from build123d import *

# Parameters (mm, degrees)
BOSS_EXTRUDE1_DEPTH                             = 15
SKETCH2_W                                       = 60
SKETCH2_H                                       = 110
BOSS_EXTRUDE2_DEPTH                             = 5
SKETCH3_R                                       = 1.25
BOSS_EXTRUDE3_DEPTH                             = 4
SKETCH4_R                                       = 1.405
BOSS_EXTRUDE4_DEPTH                             = 1
CHAMFER1_SIZE                                   = 0.5
SKETCH5_W                                       = 1
SKETCH5_H                                       = 3.260897444
CUT_EXTRUDE1_DEPTH                              = 4
SKETCH7_R                                       = 1.25
BOSS_EXTRUDE5_DEPTH                             = 4
SKETCH8_R                                       = 1.405
BOSS_EXTRUDE6_DEPTH                             = 1
CHAMFER2_SIZE                                   = 0.5
SKETCH9_W                                       = 1
SKETCH9_H                                       = 4.099421272
SKETCH9_H_2                                     = 4.814063164
CUT_EXTRUDE2_DEPTH                              = 4
SKETCH10_R                                      = 1.25
BOSS_EXTRUDE7_DEPTH                             = 4
SKETCH11_R                                      = 1.405
BOSS_EXTRUDE8_DEPTH                             = 1
CHAMFER3_SIZE                                   = 0.5
SKETCH12_W                                      = 1
SKETCH12_H                                      = 3.78691003
CUT_EXTRUDE3_DEPTH                              = 4
SKETCH14_W                                      = 27
SKETCH14_H                                      = 64
BOSS_EXTRUDE9_DEPTH                             = 5
CUT_EXTRUDE6_DEPTH                              = 85.858706094
SKETCH15_R                                      = 1
BOSS_EXTRUDE10_DEPTH                            = 4
SKETCH16_R                                      = 1.175
BOSS_EXTRUDE11_DEPTH                            = 1
CHAMFER4_SIZE                                   = 0.5
SKETCH17_W                                      = 1
SKETCH17_H                                      = 3.189279986
CUT_EXTRUDE7_DEPTH                              = 4
SKETCH20_R                                      = 1
BOSS_EXTRUDE12_DEPTH                            = 4
SKETCH21_R                                      = 1.405
BOSS_EXTRUDE13_DEPTH                            = 1
CHAMFER5_SIZE                                   = 0.5
SKETCH23_W                                      = 1
SKETCH23_H                                      = 4.222684002
CUT_EXTRUDE8_DEPTH                              = 4
CUT_EXTRUDE9_DEPTH                              = 82.547532152
SKETCH26_W                                      = 5
SKETCH26_H                                      = 5
BOSS_EXTRUDE15_DEPTH                            = 30
BOSS_EXTRUDE16_DEPTH                            = 5
CSK_FOR_M4_FLAT_HEAD_MACHINE_SCREW2_D           = 4.5
CSK_FOR_M4_FLAT_HEAD_MACHINE_SCREW2_DEPTH       = 5
CSK_FOR_M4_FLAT_HEAD_MACHINE_SCREW2_CSINK_D     = 9.4
CSK_FOR_M4_FLAT_HEAD_MACHINE_SCREW2_CSINK_ANGLE = 90
CSK_FOR_M4_FLAT_HEAD_MACHINE_SCREW2_TIP         = 1.351936393


with BuildPart() as part:
    # Sketch1 → Boss-Extrude1 (new, symmetric)
    with BuildSketch(Plane.XY):
        Polygon((0, 0), (10, 0), (55, 2.358350068), (54.738678842, 7.344654806), (10, 5), (5, 5), (5, 24), (60, 24), (60, 29), (0, 29), align=None)
    extrude(amount=BOSS_EXTRUDE1_DEPTH, both=True)

    # Sketch2 → Boss-Extrude2 (add)
    with BuildSketch(Plane(origin=(0, 29, 0), x_dir=(1, 0, 0), z_dir=(0, 1, 0))):
        with Locations((30, 0)):
            Rectangle(SKETCH2_W, SKETCH2_H)
    extrude(amount=-BOSS_EXTRUDE2_DEPTH)

    # Sketch3 → Boss-Extrude3 (add)
    with BuildSketch(Plane(origin=(0, 29, 0), x_dir=(1, 0, 0), z_dir=(0, 1, 0))):
        with Locations(Location((54, -37, 0), (0, 0, 90))):
            Circle(SKETCH3_R)
    extrude(amount=BOSS_EXTRUDE3_DEPTH)

    # Sketch4 → Boss-Extrude4 (add)
    with BuildSketch(Plane(origin=(0, 33, 0), x_dir=(1, 0, 0), z_dir=(0, 1, 0))):
        with Locations(Location((54, -37, 0), (0, 0, 270))):
            Circle(SKETCH4_R)
    extrude(amount=BOSS_EXTRUDE4_DEPTH)

    # Chamfer1
    chamfer1_edges = [part.edges().sort_by_distance(p)[0] for p in [
        (54, 34, 35.595),
    ]]
    chamfer(chamfer1_edges, length=CHAMFER1_SIZE)

    # Sketch5 → Cut-Extrude1 (cut)
    with BuildSketch(Plane(origin=(0, 34, 0), x_dir=(1, 0, 0), z_dir=(0, 1, 0))):
        with Locations((54, -37)):
            Rectangle(SKETCH5_W, SKETCH5_H)
    extrude(amount=-CUT_EXTRUDE1_DEPTH, mode=Mode.SUBTRACT)

    # Sketch7 → Boss-Extrude5 (add)
    with BuildSketch(Plane(origin=(0, 29, 0), x_dir=(1, 0, 0), z_dir=(0, 1, 0))):
        with Locations(Location((54.3, 46, 0), (0, 0, 90))):
            Circle(SKETCH7_R)
        with Locations(Location((5.7, 40, 0), (0, 0, 90))):
            Circle(SKETCH7_R)
    extrude(amount=BOSS_EXTRUDE5_DEPTH)

    # Sketch8 → Boss-Extrude6 (add)
    with BuildSketch(Plane(origin=(0, 33, 0), x_dir=(1, 0, 0), z_dir=(0, 1, 0))):
        with Locations(Location((5.7, 40, 0), (0, 0, 270))):
            Circle(SKETCH8_R)
        with Locations(Location((54.3, 46, 0), (0, 0, 270))):
            Circle(SKETCH8_R)
    extrude(amount=BOSS_EXTRUDE6_DEPTH)

    # Chamfer2
    chamfer2_edges = [part.edges().sort_by_distance(p)[0] for p in [
        (5.7, 34, -41.405),
        (54.3, 34, -47.405),
    ]]
    chamfer(chamfer2_edges, length=CHAMFER2_SIZE)

    # Sketch9 → Cut-Extrude2 (cut)
    with BuildSketch(Plane(origin=(0, 34, 0), x_dir=(1, 0, 0), z_dir=(0, 1, 0))):
        with Locations((5.7, 40)):
            Rectangle(SKETCH9_W, SKETCH9_H)
        with Locations((54.3, 46)):
            Rectangle(SKETCH9_W, SKETCH9_H_2)
    extrude(amount=-CUT_EXTRUDE2_DEPTH, mode=Mode.SUBTRACT)

    # Sketch10 → Boss-Extrude7 (add)
    with BuildSketch(Plane(origin=(0, 29, 0), x_dir=(1, 0, 0), z_dir=(0, 1, 0))):
        with Locations(Location((6, -35, 0), (0, 0, 90))):
            Circle(SKETCH10_R)
    extrude(amount=BOSS_EXTRUDE7_DEPTH)

    # Sketch11 → Boss-Extrude8 (add)
    with BuildSketch(Plane(origin=(0, 33, 0), x_dir=(1, 0, 0), z_dir=(0, 1, 0))):
        with Locations(Location((6, -35, 0), (0, 0, 270))):
            Circle(SKETCH11_R)
    extrude(amount=BOSS_EXTRUDE8_DEPTH)

    # Chamfer3
    chamfer3_edges = [part.edges().sort_by_distance(p)[0] for p in [
        (6, 34, 33.595),
    ]]
    chamfer(chamfer3_edges, length=CHAMFER3_SIZE)

    # Sketch12 → Cut-Extrude3 (cut)
    with BuildSketch(Plane(origin=(0, 34, 0), x_dir=(1, 0, 0), z_dir=(0, 1, 0))):
        with Locations((6, -35)):
            Rectangle(SKETCH12_W, SKETCH12_H)
    extrude(amount=-CUT_EXTRUDE3_DEPTH, mode=Mode.SUBTRACT)

    # Sketch14 → Boss-Extrude9 (add)
    with BuildSketch(Plane(origin=(0, 29, 0), x_dir=(1, 0, 0), z_dir=(0, 1, 0))):
        with Locations((-13.5, 23)):
            Rectangle(SKETCH14_W, SKETCH14_H)
    extrude(amount=-BOSS_EXTRUDE9_DEPTH)

    # Sketch13 → Cut-Extrude6 (cut, through all)
    with BuildSketch(Plane.XZ.offset(-24)):
        Polygon((0, 15), (0, -15), (0, -55), (60, -55), (60, 55), (0, 55), align=None)
    extrude(amount=CUT_EXTRUDE6_DEPTH, mode=Mode.SUBTRACT)

    # Sketch15 → Boss-Extrude10 (add)
    with BuildSketch(Plane(origin=(0, 29, 0), x_dir=(1, 0, 0), z_dir=(0, 1, 0))):
        with Locations(Location((-23, -6.2, 0), (0, 0, 90))):
            Circle(SKETCH15_R)
        with Locations(Location((-4, -6.2, 0), (0, 0, 90))):
            Circle(SKETCH15_R)
    extrude(amount=BOSS_EXTRUDE10_DEPTH)

    # Sketch16 → Boss-Extrude11 (add)
    with BuildSketch(Plane(origin=(0, 33, 0), x_dir=(1, 0, 0), z_dir=(0, 1, 0))):
        with Locations(Location((-23, -6.2, 0), (0, 0, 270))):
            Circle(SKETCH16_R)
        with Locations(Location((-4, -6.2, 0), (0, 0, 270))):
            Circle(SKETCH16_R)
    extrude(amount=BOSS_EXTRUDE11_DEPTH)

    # Chamfer4
    chamfer4_edges = [part.edges().sort_by_distance(p)[0] for p in [
        (-23, 34, 5.025),
        (-4, 34, 5.025),
    ]]
    chamfer(chamfer4_edges, length=CHAMFER4_SIZE)

    # Sketch17 → Cut-Extrude7 (cut)
    with BuildSketch(Plane(origin=(0, 34, 0), x_dir=(1, 0, 0), z_dir=(0, 1, 0))):
        with Locations((-23, -6.2)):
            Rectangle(SKETCH17_W, SKETCH17_H)
        with Locations((-4, -6.2)):
            Rectangle(SKETCH17_W, SKETCH17_H)
    extrude(amount=-CUT_EXTRUDE7_DEPTH, mode=Mode.SUBTRACT)

    # Sketch20 → Boss-Extrude12 (add)
    with BuildSketch(Plane(origin=(0, 29, 0), x_dir=(1, 0, 0), z_dir=(0, 1, 0))):
        with Locations(Location((-23, 50.3, 0), (0, 0, 90))):
            Circle(SKETCH20_R)
        with Locations(Location((-4, 50.3, 0), (0, 0, 90))):
            Circle(SKETCH20_R)
    extrude(amount=BOSS_EXTRUDE12_DEPTH)

    # Sketch21 → Boss-Extrude13 (add)
    with BuildSketch(Plane(origin=(0, 33, 0), x_dir=(1, 0, 0), z_dir=(0, 1, 0))):
        with Locations(Location((-23, 50.3, 0), (0, 0, 270))):
            Circle(SKETCH21_R)
        with Locations(Location((-4, 50.3, 0), (0, 0, 270))):
            Circle(SKETCH21_R)
    extrude(amount=BOSS_EXTRUDE13_DEPTH)

    # Chamfer5
    chamfer5_edges = [part.edges().sort_by_distance(p)[0] for p in [
        (-23, 34, -51.705),
        (-4, 34, -51.705),
    ]]
    chamfer(chamfer5_edges, length=CHAMFER5_SIZE)

    # Sketch23 → Cut-Extrude8 (cut)
    with BuildSketch(Plane(origin=(0, 34, 0), x_dir=(1, 0, 0), z_dir=(0, 1, 0))):
        with Locations((-23, 50.3)):
            Rectangle(SKETCH23_W, SKETCH23_H)
        with Locations((-4, 50.3)):
            Rectangle(SKETCH23_W, SKETCH23_H)
    extrude(amount=-CUT_EXTRUDE8_DEPTH, mode=Mode.SUBTRACT)

    # Sketch18 → Cut-Extrude9 (cut, through all)
    with BuildSketch(Plane(origin=(0, 29, 0), x_dir=(1, 0, 0), z_dir=(0, 1, 0))):
        Polygon((-22, 45.3), (0.7, 45.3), (0.7, 35), (10.7, 35), (10.7, 50), (49.3, 50), (49.3, 41), (55, 41), (55, -32), (49, -32), (49, -42), (55, -42), (55, -50), (6, -50), (6, -40), (11, -40), (11, -30), (5, -30), (5, -1.2), (-22, -1.2), align=None)
    extrude(amount=-CUT_EXTRUDE9_DEPTH, mode=Mode.SUBTRACT)

    # Sketch26 → Boss-Extrude15 (add)
    with BuildSketch(Plane.XZ.offset(-24)):
        with Locations((2.5, 52.5)):
            Rectangle(SKETCH26_W, SKETCH26_H)
        with Locations((57.5, 52.5)):
            Rectangle(SKETCH26_W, SKETCH26_H)
        with Locations((57.5, -52.5)):
            Rectangle(SKETCH26_W, SKETCH26_H)
        with Locations((-24.5, -52.5)):
            Rectangle(SKETCH26_W, SKETCH26_H)
        with Locations((-24.5, 6.5)):
            Rectangle(SKETCH26_W, SKETCH26_H)
    extrude(amount=BOSS_EXTRUDE15_DEPTH)

    # Sketch27 → Boss-Extrude16 (add)
    with BuildSketch(Plane.XZ.offset(6)):
        Polygon((0, 55), (60, 55), (60, -55), (0, -55), (-27, -55), (-27, 9), (0, 9), align=None)
    extrude(amount=BOSS_EXTRUDE16_DEPTH)

    # CSK for M4 Flat Head Machine Screw2
    with Locations(Plane(origin=(0, -6, 0), x_dir=(1, 0, 0), z_dir=(0, 1, 0))):
        with Locations((-13.5, 21.5), (30, 21.5), (30, -25)):
            CounterSinkHole(CSK_FOR_M4_FLAT_HEAD_MACHINE_SCREW2_D / 2, CSK_FOR_M4_FLAT_HEAD_MACHINE_SCREW2_CSINK_D / 2, depth=CSK_FOR_M4_FLAT_HEAD_MACHINE_SCREW2_DEPTH, counter_sink_angle=CSK_FOR_M4_FLAT_HEAD_MACHINE_SCREW2_CSINK_ANGLE)
            with Locations((0, 0, -(CSK_FOR_M4_FLAT_HEAD_MACHINE_SCREW2_DEPTH + CSK_FOR_M4_FLAT_HEAD_MACHINE_SCREW2_TIP / 2))):  # 118° drill point
                Cone(0, CSK_FOR_M4_FLAT_HEAD_MACHINE_SCREW2_D / 2, CSK_FOR_M4_FLAT_HEAD_MACHINE_SCREW2_TIP, mode=Mode.SUBTRACT)


solid = part.part
Geometry: final body of the model. Coordinates: model frame, mm. A direction names the side the tool comes from. Give positions to 0.01 mm unless a question says otherwise; leave off trailing zeros. Write each loop counter-clockwise with the first axis right and the second up, starting at its lowest first coordinate (ties: lowest second). Pieces come first, ordered by that corner, then holes.
(1) Cut plane A-A, the plane z = 19. Return loops of the section in (x, y), then the cut area to 3 significant figures.
(2) Access query for faces 1 (the flat face through (53.5, 32, 37)), 2 (the cylindrical face through (6.76, 30.97, 35.99)), 3 (the flat face through (11, 27, 35)). Directions: +Z, -Z, +X, -X, +Y, -Y. A direction counts if a zero-diameter tool reaches every point of the face in a straight line with its end or side. Return the directions, or none.
(3) Mould query, pull axis Y, two halves, no side actions, for faces 4 (the flat face through (27, -11, 1)), 5 (the cylindrical face through (4.855, 30.972, -39.079)), 6 (the flat face through (53.8, 32, -46)), 7 (the conical face through (27.81, -8.33, 25.91)). Classes: released by +Y, released by -Y, zero draft, split by the parting line, or undercut.
(4) Ray query, line 1 (X direction, y = -9.35, z = -21.5); line 2 (Y direction, x = 8, z = -36); line 3 (X direction, y = -10, z = 25). Return the intervals inside material, ascending.
(5) Cut plane C-C, the plane x = -13.5. Return loops of the section in (y, z).
(6) First-contact query: P1, Ø0.8, axis at y = 32, z = -50.5, coming from the -X side; P2, Ø0.8, axis at x = -23, z = -50, coming from the +Y side; P3, Ø3, axis at y = -3.5, z = 10, coming from the +X side. Flat tips, straight axial feed; report the tip coordinate or a pass-through.
(7) Cut plane D-D, the plane y = 19.5. Return loops of the section in (x, z).
(8) Cut plane B-B, the plane z = -21.5. Return loops of the section in (x, y), then the cut area to 3 significant figures.
Values follow:
1. outline: (0, -11) - (60, -11) - (60, -6) - (0, -6) - close; (0, 24) - (5, 24) - (5, 29) - (0, 29) - close; (55, 24) - (60, 24) - (60, 29) - (55, 29) - close
1. area: 350 mm2
2. face 1: +Z, +Y
2. face 2: none
2. face 3: +Y
3. face 4: released by -Y
3. face 5: undercut
3. face 6: zero draft
3. face 7: released by +Y
4. line 1: x = -27 to -15.75, -11.25 to 27.75, 32.25 to 60
4. line 2: y = -11 to -6, 24 to 29
4. line 3: x = 0 to 27.75, 32.25 to 60
5. outline: (-11, -55) - (-6, -55) - (-6, -26.2) - (-8.45, -23.75) - (-11, -23.75) - close; (-11, -19.25) - (-8.45, -19.25) - (-6, -16.8) - (-6, 9) - (-11, 9) - close; (24, -55) - (29, -55) - (29, -45.3) - (24, -45.3) - close; (24, 1.2) - (29, 1.2) - (29, 9) - (24, 9) - close
6. P1: stops at x = -24
6. P2: stops at y = 30
6. P3: stops at x = -22
7. outline: (-27, -55) - (-22, -55) - (-22, -50) - (-27, -50) - close; (-27, 4) - (-22, 4) - (-22, 9) - (-27, 9) - close; (0, 50) - (5, 50) - (5, 55) - (0, 55) - close; (55, -55) - (60, -55) - (60, -50) - (55, -50) - close; (55, 50) - (60, 50) - (60, 55) - (55, 55) - close
8. outline: (-27, -11) - (-15.75, -11) - (-15.75, -8.45) - (-18.2, -6) - (-27, -6) - close; (-27, 24) - (-22, 24) - (-22, 29) - (-27, 29) - close; (-11.25, -11) - (27.75, -11) - (27.75, -8.45) - (25.3, -6) - (-8.8, -6) - (-11.25, -8.45) - close; (32.25, -11) - (60, -11) - (60, -6) - (34.7, -6) - (32.25, -8.45) - close; (55, 24) - (60, 24) - (60, 29) - (55, 29) - close
8. area: 428 mm2
